Part model, mm, in its own coordinate system. Face numbers are marked on the shaded views. A direction names the side the tool comes from. Round coordinates to 2 decimals unless told otherwise and drop trailing zeros. Write each loop counter-clockwise with the first axis right and the second up, starting at its lowest first coordinate (ties: lowest second). Pieces come first, ordered by that corner, then holes. Notation, with made-up numbers: (-7.5, 65) -> (17.5, 65) arc R15 ccw to (17.5, 76) -> close; hole circle Ø9 at (11, 3). An arc over 180 degrees is marked (long way). Return JSON: item names as keys, results as strings. Group by question number.
(1) Mould opens along X. For the marked faces 1, 2 and 3 say: +X half, -X half, draft (parallel to the pull), parting line (faces both ways), or undercut.
(2) Saw through at C-C (z = -6.25). List the corners of the cut face in (x, y).
(3) Saw through at D-D (x = -7). List the corners of the cut face in (y, z).
(4) Tool access for the marked faces 4, 5 and 6: list every direction of +Z, -Z, +X, -X, +Y, -Y with a clear straight run to the whole face (end or side of a thin tool).
(5) Drop flat-ended pins along their axis: pin 1 Ø7 at (x, z) = (-20, -10) entering from -Y; pin 2 Ø6 at (x, z) = (-21.5, -11.5) entering from +Y; pin 3 Ø3.5 at (x, z) = (-40, -10) entering from -Y. Give the stop position or say it passes through.
(6) Saw through at B-B (y = -15). List the corners of the cut face in (x, z), plus the area to 3 significant figures.
(7) Drill centre lines: L1, parallel to Z at x = -20, y = -14.5; L2, parallel to Z at x = -40, y = -5; L3, parallel to X at y = -4, z = -10. Where is each one in solid material? Low to high. Write a range as from..to.
(8) Saw through at A-A (x = -20). List the corners of the cut face in (y, z), plus the area to 3 significant figures.
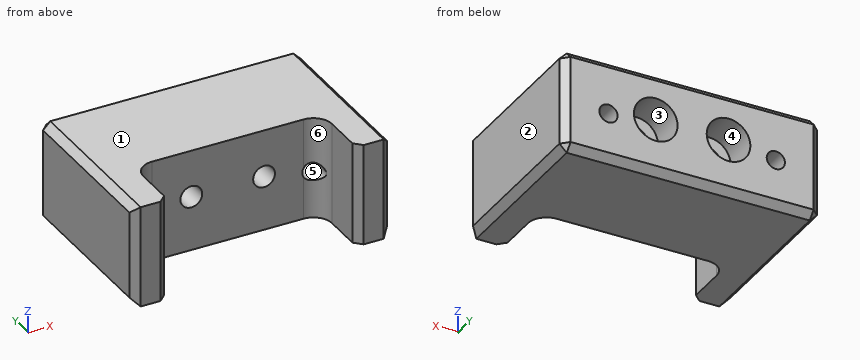
Autodesk Inventor part; units mm, degrees
ref_plane "Work Plane3" through (-49.05, -33.575, -1214.2) normal (0, -1, 0) x (1, 0, 0)
ref_plane "YZ Plane" through (0, 0, 0) normal (1, 0, 0) x (0, 1, 0)
ref_plane "XZ Plane" through (0, 0, 0) normal (0, 1, 0) x (-1, 0, 0)
sketch "Sketch1" plane through (0, 0, 0) normal (0, 1, 0) x (-1, 0, 0)
  line L0 (0, 0) -> (60, 0) construction
  line L1 (60, 0) -> (60, -20) construction
  line L2 (60, -20) -> (0, -20) construction
  line L3 (0, -20) -> (0, 0) construction
  line L4 (60.5, 0.5) -> (-0.5, 0.5)
  line L5 (-0.5, 0.5) -> (-0.5, -20.5)
  line L6 (-0.5, -20.5) -> (60.5, -20.5)
  line L7 (60.5, -20.5) -> (60.5, 0.5)
  circle A0 centre (53, -12) radius 2.5
  circle A1 centre (7, -12) radius 2.5
  line L8 (53, -12) -> (7, -12) construction
  point P0 (30, -12)
  point P1 (30, -20)
  point P2 (0, -10)
  point P3 (-0.5, -10)
  dimension "d0" = 20
  dimension "d1" = 60
  dimension "d2" = 0.5
  dimension "d3" = 0.5
  dimension "d4" = 0.5
  dimension "d5" = 0.5
  dimension "d6" = 5
  dimension "d7" = 46
  dimension "d109" = 2
sketch "Sketch2" plane through (0, 0, 0) normal (0, 1, 0) x (-1, 0, 0)
  line L0 (-5.4, 5) -> (65.4, 5)
  line L1 (65.4, 5) -> (65.4, -25)
  line L2 (65.4, -25) -> (-5.4, -25)
  line L3 (-5.4, -25) -> (-5.4, 5)
  line L4 (60.5, -20.5) -> (60.5, 0.5) construction
  line L5 (-0.5, 0.5) -> (-0.5, -20.5) construction
  line L6 (-0.5, -20.5) -> (60.5, -20.5) construction
  point P0 (0, 0)
  point P1 (60.5, -10)
  point P2 (65.4, -10)
  point P3 (30, -20.5)
  point P4 (30, -25)
  dimension "d9" = 70.8
  dimension "d10" = 30
  dimension "d44" = 35.4
extrude "Extrusion1" add sketch "Sketch2" against normal blind 30.4
extrude "Extrusion3" cut sketch "Sketch1" against normal blind 43.3375 and the other way blind 30.4 contours A0 | A1
sketch "Sketch3" plane through (5.4, -30.4, -25) normal (0, 0, -1) x (1, 0, 0)
  line L0 (-70.8, 0) -> (0, 0)
  line L1 (0, 0) -> (0, 17.5)
  line L2 (0, 17.5) -> (-9.5, 17.5)
  line L3 (-9.5, 17.5) -> (-9.5, 5.08)
  line L4 (-14.58, 0) -> (-56.22, 0)
  line L5 (-61.3, 5.08) -> (-61.3, 17.5)
  line L6 (-61.3, 17.5) -> (-70.8, 17.5)
  line L7 (-70.8, 17.5) -> (-70.8, 0)
  arc A0 (-14.58, 0) -> (-9.5, 5.08) centre (-14.58, 5.08) ccw
  arc A1 (-61.3, 5.08) -> (-56.22, 0) centre (-56.22, 5.08) ccw
  point P0 (-9.5, 0)
  point P1 (-61.3, 0)
  point P2 (-61.3, 11.29)
  point P3 (-9.5, 11.29)
  point P4 (-4.75, 17.5)
  dimension "d94" = 51.8
  dimension "d95" = 17.5
  dimension "d96" = 5.08
extrude "Extrusion4" add sketch "Sketch3" against normal up to surface (30 mm away)
ref_plane "Work Plane3" through (-49.05, -33.575, -1214.2) normal (0, -1, 0) x (1, 0, 0)
sketch "Sketch4" plane through (0, 0, 0) normal (0, 1, 0) x (1, 0, 0)
  line L0 (-60.5, 20.5) -> (0.5, 20.5) construction
  line L1 (-60.5, -0.5) -> (-60.5, 20.5) construction
  circle A0 centre (-40, 10) radius 3
  line L2 (5.4, 25) -> (-65.4, 25)
  line L3 (-65.4, 25) -> (-65.4, -5)
  circle A1 centre (-20, 10) radius 3
  line L4 (-40, 10) -> (-20, 10) construction
  point P0 (0, 0)
  point P1 (-30, 20.5)
  point P2 (-60.5, 10)
  point P3 (-65.4, 20.5)
  point P4 (5.4, 20.5)
  point P5 (-30, 20.5)
  point P6 (-60.5, 10)
  point P7 (-65.4, 10)
  point P8 (-30, 25)
  point P9 (-30, 10)
  dimension "d82" = 6
  dimension "d98" = 20
  dimension "d107" = 0
extrude "Extrusion5" cut sketch "Sketch4" against normal up to surface (33.575 mm away)
extrude "Extrusion2" cut sketch "Sketch1" against normal blind 43.3375 and the other way blind 5 contours A0 | A1
sketch "Sketch8" plane through (15.4, 40, -25) normal (0, 0, -1) x (1, 0, 0)
  line L0 (25.4, 30) -> (34.4, 30)
  line L1 (34.4, 30) -> (35.4, 31)
  line L2 (35.4, 31) -> (35.4, 34)
  line L3 (35.4, 34) -> (31.95, 37.45)
  line L4 (31.95, 37.45) -> (31.95, 39.8767)
  line L5 (31.95, 39.8767) -> (33.1672, 41.0939)
  arc A0 (34.8792, 42.8058) -> (33.1672, 41.0939) centre (35.1489, 40.8241) ccw
  line L6 (34.8792, 42.8058) -> (35.4, 43.3267)
  line L7 (35.4, 43.3267) -> (35.4, 44.66)
  line L8 (35.4, 44.66) -> (34.8792, 45.1808)
  arc A1 (33.1672, 46.8928) -> (34.8792, 45.1808) centre (35.1489, 47.1626) ccw
  line L9 (33.1672, 46.8928) -> (32.56, 47.5)
  line L10 (32.56, 47.5) -> (25.4, 47.5)
  line L11 (25.4, 47.5) -> (25.4, 30) construction
  line L12 (33.1672, 41.0939) -> (34.8792, 42.8058) construction
  line L13 (33.1672, 46.8928) -> (34.8792, 45.1808) construction
  line L14 (25.4, 30) -> (16.4, 30)
  line L15 (16.4, 30) -> (15.4, 31)
  line L16 (15.4, 31) -> (15.4, 34)
  line L17 (15.4, 34) -> (18.85, 37.45)
  line L18 (18.85, 37.45) -> (18.85, 39.8767)
  line L19 (18.85, 39.8767) -> (17.6328, 41.0939)
  arc A2 (17.6328, 41.0939) -> (15.9208, 42.8058) centre (15.6511, 40.8241) ccw
  line L20 (15.9208, 42.8058) -> (15.4, 43.3267)
  line L21 (15.4, 43.3267) -> (15.4, 44.66)
  line L22 (15.4, 44.66) -> (15.9208, 45.1808)
  arc A3 (15.9208, 45.1808) -> (17.6328, 46.8928) centre (15.6511, 47.1626) ccw
  line L23 (17.6328, 46.8928) -> (18.24, 47.5)
  line L24 (18.24, 47.5) -> (25.4, 47.5)
  line L25 (17.6328, 41.0939) -> (15.9208, 42.8058) construction
  line L26 (17.6328, 46.8928) -> (15.9208, 45.1808) construction
  arc A4 (50.8, 26.825) -> (47.625, 30) centre (47.625, 26.825) ccw construction
  line L27 (34.4, 30) -> (35.4, 30)
  line L28 (3.175, 30) -> (47.625, 30)
  line L29 (35.4, 31) -> (35.4, 30)
  line L30 (15.4, 31) -> (15.4, 30)
  line L31 (15.4, 30) -> (16.4, 30)
  point P0 (-15.4, 40)
  point P1 (35.4, 32.5)
  dimension "d64" = 1
  dimension "d65" = 3
  dimension "d66" = 135
  dimension "d67" = 2
  dimension "d69" = 3.45
  dimension "d71" = 17.5
  dimension "d72" = 7.16
  dimension "d73" = 2.375
  dimension "d74" = 1.3333
  dimension "d75" = 2.4211
  dimension "d76" = 15.4
  dimension "d77" = 10
extrude "Extrusion8" [suppressed]
thicken "Thicken1" [suppressed]
sketch "Sketch11" plane through (0, 0, 0) normal (0, 1, 0) x (1, 0, 0)
  circle A0 centre (-20, 10) radius 6
  circle A1 centre (-40, 10) radius 3
  circle A2 centre (-20, 10) radius 3
  circle A3 centre (-40, 10) radius 6
  point P0 (0, 0)
  dimension "d99" = 12
extrude "Extrusion11" cut sketch "Sketch11" against normal blind 10 contours A0 | A1 | A2 | A3
sketch "Sketch12" plane through (-50.82, -30.4, 5) normal (0, 0, 1) x (1, 0, 0)
  line L0 (-31.8767, 47.5596) -> (80.4706, 47.5596)
  line L1 (80.4706, 47.5596) -> (80.4706, -43.9783)
  line L2 (80.4706, -43.9783) -> (-31.8767, -43.9783)
  line L3 (-31.8767, -43.9783) -> (-31.8767, 47.5596)
  point P0 (50.82, 30.4)
extrude "Extrusion12" cut sketch "Sketch12" against normal blind 2
chamfer "Chamfer1" distance 2 angle 45 12 edges at (5.4, 0, -11) (-30, 0, -25) (5.4, -23.95, -25) (-65.4, -23.95, -25) (-55.9, -47.9, -11) (5.4, -47.9, -11) (-65.4, 0, -11) (-65.4, -47.9, -11) (-4.1, -47.9, -11) (-30, 0, 3) (-65.4, -23.95, 3) (5.4, -23.95, 3)
properties part number "BK12_Spacer"
Computed values:
{
 "1": {"face 1": "draft", "face 2": "+X half", "face 3": "undercut"},
 "2": {"outline": "(-65.4, -45.9) -> (-63.4, -47.9) -> (-57.9, -47.9) -> (-55.9, -45.9) -> (-55.9, -35.48) arc R5.08 cw to (-50.82, -30.4) -> (-9.18, -30.4) arc R5.08 cw to (-4.1, -35.48) -> (-4.1, -45.9) -> (-2.1, -47.9) -> (3.4, -47.9) -> (5.4, -45.9) -> (5.4, -2) -> (3.4, 0) -> (-15.32, 0) -> (-15.32, -10) -> (-24.68, -10) -> (-24.68, 0) -> (-35.32, 0) -> (-35.32, -10) -> (-44.68, -10) -> (-44.68, 0) -> (-63.4, 0) -> (-65.4, -2) -> close"},
 "3": {"outline": "(-30.89, -25) -> (-2, -25) -> (0, -23) -> (0, -14.5) -> (-30.89, -14.5) -> close; (-30.89, -9.5) -> (0, -9.5) -> (0, 1) -> (-2, 3) -> (-30.89, 3) -> close"},
 "4": {"face 4": "+Y", "face 5": "+Y, -Y", "face 6": "+Z, -Z, -Y"},
 "5": {"pin 1": "y = -30.4", "pin 2": "y = -10", "pin 3": "through"},
 "6": {"outline": "(-65.4, -23) -> (-63.4, -25) -> (3.4, -25) -> (5.4, -23) -> (5.4, 1) -> (3.4, 3) -> (-63.4, 3) -> (-65.4, 1) -> close; hole circle Ø5 at (-53, -12); hole circle Ø6 at (-40, -10); hole circle Ø6 at (-20, -10); hole circle Ø5 at (-7, -12)", "area": "1,880 mm2"},
 "7": {"L1": "-25..-13, -7..3", "L2": "-25..-16, -4..3", "L3": "-65.4..-54.5, -51.5..-46, -34..-26, -14..-8.5, -5.5..5.4"},
 "8": {"outline": "(-30.4, -25) -> (-2, -25) -> (0, -23) -> (0, -16) -> (-10, -16) -> (-10, -13) -> (-30.4, -13) -> close; (-30.4, -7) -> (-10, -7) -> (-10, -4) -> (0, -4) -> (0, 1) -> (-2, 3) -> (-30.4, 3) -> close", "area": "605 mm2"}
}
